Can you work these out from the model? Positions are in its coordinate system, mm. A direction names the side the tool comes from. Coordinates: 2 decimals unless noted, no trailing zeros. Write each loop counter-clockwise with the first axis right and the second up, starting at its lowest first coordinate (ties: lowest second). Pieces come first, ordered by that corner, then holes. Notation, with made-up numbers: M 42.5,39.5 L 81.5,39.5 A32 ccw 81.5,75.5 Z; hole C -38.5,61 d3. An arc over 180 degrees is marked long. Answer as a JSON object with one key per item and string values. Group by question number.
from build123d import *

# Parameters (mm, degrees)
SKETCH1_W           = 35.814
SKETCH1_H           = 7.1628
BOSS_EXTRUDE1_DEPTH = 1.524
FILLET1_R           = 2.54
FILLET2_R           = 0.127
BOSS_EXTRUDE2_DEPTH = 0.381
SKETCH5_R           = 1.2827
CUT_EXTRUDE2_DEPTH  = 2.54
SKETCH9_R           = 1.7526
CUT_EXTRUDE5_DEPTH  = 1.016
CUT_EXTRUDE6_START  = -0.381
CUT_EXTRUDE6_DEPTH  = 0.381
SKETCH17_R          = 1.7526
CUT_EXTRUDE11_DEPTH = 19.289869627
SKETCH18_R          = 1.7526
CUT_EXTRUDE12_DEPTH = 19.325109849
SKETCH19_R          = 0.381
CUT_EXTRUDE13_DEPTH = 0.127
SKETCH20_R          = 0.1905
CUT_EXTRUDE14_DEPTH = 0.762


with BuildPart() as part:
    # Sketch1 → Boss-Extrude1 (new body)
    with BuildSketch(Plane(origin=(0, 0, 0), x_dir=(1, 0, 0), z_dir=(0, 1, 0))):
        Rectangle(SKETCH1_W, SKETCH1_H)
    extrude(amount=BOSS_EXTRUDE1_DEPTH)

    # Fillet1
    fillet1_edges = [part.edges().sort_by_distance(p)[0] for p in [
        (-17.907, 0.762, -3.5814),
        (17.907, 0.762, -3.5814),
        (17.907, 0.762, 3.5814),
        (-17.907, 0.762, 3.5814),
    ]]
    fillet(fillet1_edges, radius=FILLET1_R)

    # Fillet2
    fillet2_edges = [part.edges().sort_by_distance(p)[0] for p in [
        (-17.907, 1.524, 0),
        (0, 1.524, -3.5814),
        (0, 1.524, 3.5814),
        (17.907, 1.524, 0),
        (17.163051224, 1.524, 2.837451224),
        (17.163051224, 1.524, -2.837451224),
        (-17.163051224, 1.524, 2.837451224),
        (-17.163051224, 1.524, -2.837451224),
    ]]
    fillet(fillet2_edges, radius=FILLET2_R)

    # Sketch4 → Boss-Extrude2 (add)
    with BuildSketch(Plane.XZ.offset(-0.381)):
        with BuildLine():
            Line((-15.367, 2.9464), (-15.367, 3.2004))
            ThreePointArc((-15.367, 3.2004), (-16.893643541, 2.568043541), (-17.526, 1.0414))
            Line((-17.526, 1.0414), (-17.526, -1.0414))
            ThreePointArc((-17.526, -1.0414), (-16.893643541, -2.568043541), (-15.367, -3.2004))
            Line((-15.367, -3.2004), (-15.367, -2.9464))
            ThreePointArc((-15.367, -2.9464), (-16.714038418, -2.388438418), (-17.272, -1.0414))
            Line((-17.272, -1.0414), (-17.272, 1.0414))
            ThreePointArc((-17.272, 1.0414), (-16.714038418, 2.388438418), (-15.367, 2.9464))
        make_face()
    boss_extrude2 = extrude(amount=BOSS_EXTRUDE2_DEPTH)

    # Mirror3: Boss-Extrude2 across plane
    add(boss_extrude2.mirror(Plane(origin=(0, 0, 0), x_dir=(0, 0, 1), z_dir=(1, 0, 0))))

    # Sketch5 → Cut-Extrude2 (cut)
    with BuildSketch(Plane(origin=(0, 1.524, 0), x_dir=(1, 0, 0), z_dir=(0, 1, 0))):
        with Locations(Location((-12.7762, -0.7112, 0), (0, 0, 270))):
            Circle(SKETCH5_R)
    cut_extrude2 = extrude(amount=-CUT_EXTRUDE2_DEPTH, mode=Mode.SUBTRACT)

    # Sketch9 → Cut-Extrude5 (cut)
    with BuildSketch(Plane(origin=(0, 1.524, 0), x_dir=(1, 0, 0), z_dir=(0, 1, 0))):
        with Locations(Location((-12.7762, -0.7112, 0), (0, 0, 270))):
            Circle(SKETCH9_R)
    cut_extrude5 = extrude(amount=-CUT_EXTRUDE5_DEPTH, mode=Mode.SUBTRACT)

    # Mirror4: Cut-Extrude2, Cut-Extrude5 across plane
    add(cut_extrude2.mirror(Plane(origin=(0, 0, 0), x_dir=(0, 0, 1), z_dir=(1, 0, 0))), mode=Mode.SUBTRACT)
    add(cut_extrude5.mirror(Plane(origin=(0, 0, 0), x_dir=(0, 0, 1), z_dir=(1, 0, 0))), mode=Mode.SUBTRACT)

    # Sketch10 → Cut-Extrude6 (cut)
    with BuildSketch(Plane.XZ.offset(CUT_EXTRUDE6_START)):
        with BuildLine():
            Line((17.907, 1.0414), (17.907, -1.0414))
            ThreePointArc((17.907, -1.0414), (17.163051224, -2.837451224), (15.367, -3.5814))
            Line((15.367, -3.5814), (-15.367, -3.5814))
            ThreePointArc((-15.367, -3.5814), (-17.163051224, -2.837451224), (-17.907, -1.0414))
            Line((-17.907, -1.0414), (-17.907, 1.0414))
            ThreePointArc((-17.907, 1.0414), (-17.163051224, 2.837451224), (-15.367, 3.5814))
            Line((-15.367, 3.5814), (15.367, 3.5814))
            ThreePointArc((15.367, 3.5814), (17.163051224, 2.837451224), (17.907, 1.0414))
        make_face()
        with BuildLine():
            Line((-15.367, 2.9464), (15.367, 2.9464))
            ThreePointArc((15.367, 2.9464), (16.714038418, 2.388438418), (17.272, 1.0414))
            Line((17.272, 1.0414), (17.272, -1.0414))
            ThreePointArc((17.272, -1.0414), (16.714038418, -2.388438418), (15.367, -2.9464))
            Line((15.367, -2.9464), (-15.367, -2.9464))
            ThreePointArc((-15.367, -2.9464), (-16.714038418, -2.388438418), (-17.272, -1.0414))
            Line((-17.272, -1.0414), (-17.272, 1.0414))
            ThreePointArc((-17.272, 1.0414), (-16.714038418, 2.388438418), (-15.367, 2.9464))
        make_face(mode=Mode.SUBTRACT)
    extrude(amount=CUT_EXTRUDE6_DEPTH, mode=Mode.SUBTRACT)

    # Sketch17 → Cut-Extrude11 (cut, through all)
    with BuildSketch(Plane(origin=(0, 0.508, 0), x_dir=(1, 0, 0), z_dir=(0, 1, 0))):
        with Locations(Location((-12.7762, -0.7112, 0), (0, 0, 270))):
            Circle(SKETCH17_R)
    extrude(amount=-CUT_EXTRUDE11_DEPTH, mode=Mode.SUBTRACT)

    # Sketch18 → Cut-Extrude12 (cut, through all)
    with BuildSketch(Plane(origin=(0, 1.524, 0), x_dir=(1, 0, 0), z_dir=(0, 1, 0))):
        with Locations(Location((12.7762, -0.7112, 0), (0, 0, 270))):
            Circle(SKETCH18_R)
    extrude(amount=-CUT_EXTRUDE12_DEPTH, mode=Mode.SUBTRACT)

    # Sketch19 → Cut-Extrude13 (cut)
    with BuildSketch(Plane.XZ):
        with Locations(Location((0, 0.7112, 0), (0, 0, 270))):
            Circle(SKETCH19_R)
    extrude(amount=-CUT_EXTRUDE13_DEPTH, mode=Mode.SUBTRACT)

    # Sketch20 → Cut-Extrude14 (cut)
    with BuildSketch(Plane.XZ):
        with Locations(Location((0, 0.7112, 0), (0, 0, 270))):
            Circle(SKETCH20_R)
    extrude(amount=-CUT_EXTRUDE14_DEPTH, mode=Mode.SUBTRACT)


solid = part.part
Q1. On a 3-axis mill with a long thin cutter (end or side, diameter ignored), from which of +Z, -Z, +X, -X, +Y, -Y can I reach the whole of each face in a straight line? I mean faces 1 (the cylindrical face through (-16.7, 0.2, -2.4)), 2 (the cylindrical face through (16.7, 0.2, -2.4)), 3 (the cylindrical face through (16.7, 0.2, 2.4)), 4 (the cylindrical face through (-16.7, 0.2, 2.4)). Say none if no direction works.
Q2. If we section it at B-B on y = 1.05: List the corners of the cut face in (x, z) for me, and give its area (3 significant figures).
Q3. We'd pull the mould along Z, two halves only. Please class faces 5 (the cylindrical face through (17.1, 0.9, 2.9)), 6 (the cylindrical face through (-11.04, 0.77, 0.48)), 7 (the flat face through (1.4, 0.381, -3.2)): pulls with the +Z half, pulls with the -Z half, needs draft (parallel to the pull), parting line crosses it, or undercut.
Q4. Will this pin go through, and if not, where does the flat tip stop? pin 1 (3 mm diameter, centred on x = -12.78, z = 0.71, fed in from +Y).
Q5. If we section it at A-A on z = -0.5: List the corners of the cut face in (x, y) for me.
Q6. If we section it at C-C on x = 7.5: List the corners of the cut face in (y, z) for me, and give its area (3 significant figures).
Q7. Please list where these lines run through material, in increasing order: L1, parallel to X at y = 0.55, z = 0.75; L2, parallel to X at y = 0.85, z = -0.75; L3, parallel to X at y = 0.9, z = 2.25.
Reply:
{
 "1": {"face 1": "-Z, -X, -Y", "face 2": "-Z, +X, -Y", "face 3": "+Z, +X, -Y", "face 4": "+Z, -X, -Y"},
 "2": {"outline": "M -17.91,-1.04 A2.54 ccw -15.37,-3.58 L 15.37,-3.58 A2.54 ccw 17.91,-1.04 L 17.91,1.04 A2.54 ccw 15.37,3.58 L -15.37,3.58 A2.54 ccw -17.91,1.04 Z; hole C -12.78,0.71 d3.51; hole C 12.78,0.71 d3.51", "area": "232 mm^2"},
 "3": {"face 5": "pulls with the +Z half", "face 6": "undercut", "face 7": "needs draft"},
 "4": {"pin 1": "through"},
 "5": {"outline": "M -17.91,0.38 L -17.27,0.38 L -17.27,0 L -14.04,0 L -14.04,1.52 L -17.78,1.52 A0.13 ccw -17.91,1.4 Z; M -11.51,0 L 11.51,0 L 11.51,1.52 L -11.51,1.52 Z; M 14.04,0 L 17.27,0 L 17.27,0.38 L 17.91,0.38 L 17.91,1.4 A0.13 ccw 17.78,1.52 L 14.04,1.52 Z"},
 "6": {"outline": "M 0,-2.95 L 0.38,-2.95 L 0.38,-3.58 L 1.4,-3.58 A0.13 ccw 1.52,-3.45 L 1.52,3.45 A0.13 ccw 1.4,3.58 L 0.38,3.58 L 0.38,2.95 L 0,2.95 Z", "area": "10.4 mm^2"},
 "7": {"L1": "-17.91 to -14.53, -11.02 to -0.19, 0.19 to 11.02, 14.53 to 17.91", "L2": "-17.91 to -13.74, -11.81 to 11.81, 13.74 to 17.91", "L3": "-17.6 to -13.62, -11.94 to 11.94, 13.62 to 17.6"}
}
